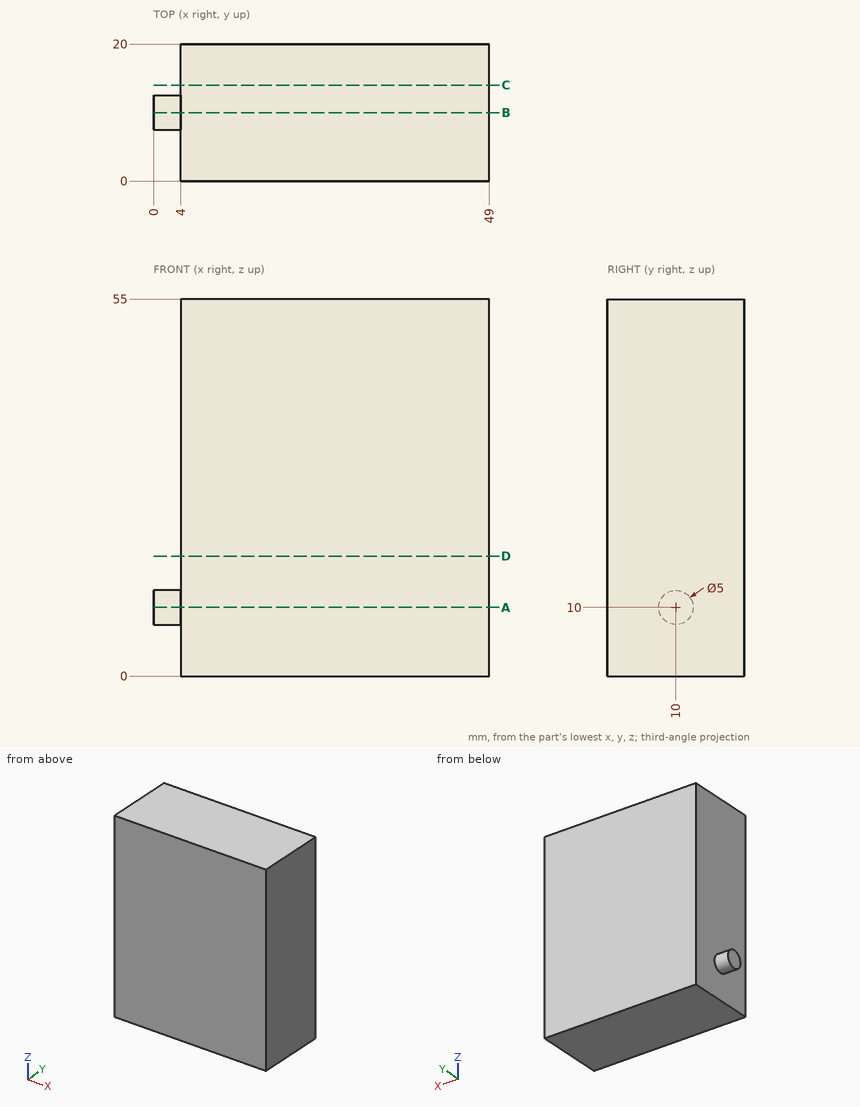
Drawing for the job (mm, zero at the part's lowest x, y, z). Give positions to 0.01 mm unless a question says otherwise; leave off trailing zeros. Order: outer loops, then holes, each group sorted by start corner. A loop starts at its lowest first (then second) coordinate and runs counter-clockwise, first axis right, second up. Notation, with made-up numbers: (52, 12) -> (106, 12) arc R17 ccw to (106, 23) -> close; hole circle Ø5 at (85, -30). An arc over 180 degrees is marked (long way). Use one line per item in the form item = value.
(1) Saw through at A-A (z = 10). Write the cut outline in (x, y), then the cut area to 3 significant figures.
Solution:
outline = (0, 7.5) -> (4, 7.5) -> (4, 0) -> (49, 0) -> (49, 20) -> (4, 20) -> (4, 12.5) -> (0, 12.5) -> close
area = 920 mm²
(2) Saw through at D-D (z = 17.5). Write the cut outline in (x, y).
Solution:
outline = (4, 0) -> (49, 0) -> (49, 20) -> (4, 20) -> close
(3) Saw through at B-B (y = 10). Write the cut outline in (x, z).
Solution:
outline = (0, 7.5) -> (4, 7.5) -> (4, 0) -> (49, 0) -> (49, 55) -> (4, 55) -> (4, 12.5) -> (0, 12.5) -> close
(4) Drill centre line: line 1 (X direction, y = 11.75, z = 52). Where is it in solid material? Low to high. Write a range as from..to.
Solution:
line_1 = 4..49
(5) Saw through at C-C (y = 14). Write the cut outline in (x, z), then the cut area to 4 significant figures.
Solution:
outline = (4, 0) -> (49, 0) -> (49, 55) -> (4, 55) -> close
area = 2,475 mm²
(6) Flat gauge pins, fed straight in: P1, Ø8, axis at y = 17, z = 35, coming from the -X side; P2, Ø12, axis at x = 6.5, z = 22.5, coming from the -Y side. Where does each tip first touch, or does it go through?
Solution:
P1 = 4
P2 = 0
